Input: part model. Units: mm. Frame: model coordinates. A direction names the side the tool comes from. Round coordinates to 2 decimals unless told otherwise and drop trailing zeros. Order: outer loops, then holes, each group sorted by start corner. A loop starts at its lowest first (then second) coordinate and runs counter-clockwise, first axis right, second up.
Item 1: Line query: L1, parallel to Y at x = 0, z = 13; L2, parallel to Z at x = -2.5, y = -15; L3, parallel to X at y = 24, z = 6.75. Output: solid intervals per line, ascending.
Item 2: Cut plane C-C on z = 7.62. Output: boundary loops of the cut face in (x, y), then the cut area to 3 significant figures.
Item 3: Cut plane D-D on z = 1.5. Output: boundary loops of the cut face in (x, y), then the cut area to 3 significant figures.
Item 4: Cut plane A-A on y = 0. Output: boundary loops of the cut face in (x, z).
Item 5: Reachability of faces 4 (the flat face through (30, 11, 0)), 5 (the cylindrical face through (-1.915, 30.412, 6.152)) from +Z, -Z, +X, -X, +Y, -Y: full face, straight path, thin tool, end or side. Return the list, or none.
Item 6: First-contact query: pin 1 (4 mm diameter, centred on x = -25, z = 9, fed in from -Y); pin 2 (17.5 mm diameter, centred on x = -3, y = 9.5, fed in from +Z); pin 3 (8 mm diameter, centred on y = 13.5, z = 11, fed in from +X); pin 4 (3.5 mm diameter, centred on x = -8.89, y = 40.83, fed in from -Z). Flat tips, straight axial feed; report the tip coordinate or a pass-through.
Item 7: Mould query, pull axis Z, two halves, no side actions, for faces 1 (the cylindrical face through (-11.01, 41.49, -2.58)), 2 (the flat face through (14, -26, 13.97)), 3 (the cylindrical face through (30.449, -1.915, 6.152)). Classes: released by +Z, released by -Z, zero draft, split by the parting line, or undercut.
```python
from build123d import *

# Parameters (mm, degrees)
F0_R      = 31.75
F0_R_2    = 29.21
F1_DEPTH  = 13.97
F4_R      = 45.974
F5_DEPTH  = 5.08
F6_R      = 2.413
F7_DEPTH  = 38.1
F9_D      = 4.445
F9_DEPTH  = 12.7
F10_R     = 2.413
F11_DEPTH = 50.8


with BuildPart() as f1:
    # F0 (on Top) → F1 (new body)
    with BuildSketch(Plane.XY):
        Circle(F0_R)
        Circle(F0_R_2, mode=Mode.SUBTRACT)
    extrude(amount=F1_DEPTH)

    # F4 (on Top) → F5 (join)
    with BuildSketch(Plane.XY):
        Circle(F4_R)
    extrude(amount=-F5_DEPTH)

    # F6 (on Front) → F7 (cut, symmetric)
    with BuildSketch(Plane.XZ):
        with Locations((0, 7.62)):
            Circle(F6_R)
    extrude(amount=F7_DEPTH, both=True, mode=Mode.SUBTRACT)

    # F9
    with Locations(Plane.XY):
        with Locations((-8.89, 40.826303), (-30.911615, -28.112117), (39.801615, -12.714185)):
            Hole(F9_D / 2, depth=F9_DEPTH)

    # F10 (on Right) → F11 (cut, symmetric)
    with BuildSketch(Plane.YZ):
        with Locations((0, 7.62)):
            Circle(F10_R)
    extrude(amount=F11_DEPTH, both=True, mode=Mode.SUBTRACT)


solid = f1.part
```
From the geometry:
1. L1: y = -31.75 to -29.21, 29.21 to 31.75
1. L2: z = -5.08 to 0
1. L3: x = -20.79 to -16.65, 16.65 to 20.79
2. outline: (-31.66, -2.41) arc R31.75 ccw to (-2.41, -31.66) - (-2.41, -29.11) arc R29.21 cw to (-29.11, -2.41) - close; (-31.66, 2.41) - (-29.11, 2.41) arc R29.21 cw to (-2.41, 29.11) - (-2.41, 31.66) arc R31.75 ccw to start; (2.41, -31.66) arc R31.75 ccw to (31.66, -2.41) - (29.11, -2.41) arc R29.21 cw to (2.41, -29.11) - close; (2.41, 29.11) arc R29.21 cw to (29.11, 2.41) - (31.66, 2.41) arc R31.75 ccw to (2.41, 31.66) - close
2. area: 437 mm2
3. outline: circle Ø63.5 at (0, 0); hole circle Ø58.42 at (0, 0)
3. area: 486 mm2
4. outline: (-45.97, -5.08) - (45.97, -5.08) - (45.97, 0) - (31.75, 0) - (31.75, 5.21) - (29.21, 5.21) - (29.21, 0) - (-29.21, 0) - (-29.21, 5.21) - (-31.75, 5.21) - (-31.75, 0) - (-45.97, 0) - close; (-31.75, 10.03) - (-29.21, 10.03) - (-29.21, 13.97) - (-31.75, 13.97) - close; (29.21, 10.03) - (31.75, 10.03) - (31.75, 13.97) - (29.21, 13.97) - close
5. face 4: +Z
5. face 5: +Y, -Y
6. pin 1: stops at y = -21.89
6. pin 2: stops at z = 0
6. pin 3: stops at x = 30.3
6. pin 4: passes through
7. face 1: zero draft
7. face 2: released by +Z
7. face 3: undercut
